Geometry check sheet. Reference: the model listing, model coordinates, mm. Face numbers are marked on the shaded views. A direction names the side the tool comes from. Round coordinates to 2 decimals unless told otherwise and drop trailing zeros. Order: outer loops, then holes, each group sorted by start corner. A loop starts at its lowest first (then second) coordinate and runs counter-clockwise, first axis right, second up.
(1) Release check for a two-part mould opening along Z. For the marked faces 3, 4 and 5 record: +Z half, -Z half, draft (parallel to the pull), parting line (faces both ways), or undercut.
(2) Set-up check for the marked faces 1 and 2: record each of +Z, -Z, +X, -X, +Y, -Y from which the full face is reachable in a straight line by a thin tool's end or side.
(3) Sectioned sample at D-D (x = 30). Record the boundary of the cut face in (y, z).
(4) Sectioned sample at B-B (x = -54). Record the boundary of the cut face in (y, z), plus the area to 3 significant figures.
(5) Sectioned sample at C-C (z = -28.5). Record the boundary of the cut face in (x, y), plus the area to 3 significant figures.
(6) Material ranges on line 1 along Y through (x, z) = (54, -37.65); line 2 along Z through (x, y) = (-28.5, 15.5); line 3 along X through (y, z) = (15.5, 10.5), recorded low to high.
(7) Go/stop test with flat-tipped pins: pin 1 (10 mm diameter, centred on x = 6, z = -13.5, fed in from +Y); pin 2 (6.5 mm diameter, centred on y = 11.5, z = 4, fed in from +X); pin 3 (3 mm diameter, centred on x = -38.5, z = -29, fed in from +Y). Record where each tip stops, or that it passes through.
(8) Sectioned sample at A-A (y = 22). Record the boundary of the cut face in (x, z), plus the area to 3 significant figures.
from build123d import *

# Parameters (mm, degrees)
SKETCH1_W           = 100
SKETCH1_H           = 80
BOSS_EXTRUDE1_DEPTH = 3
SKETCH2_W           = 100
SKETCH2_H           = 80
SKETCH2_W_2         = 97
SKETCH2_H_2         = 77
BOSS_EXTRUDE2_DEPTH = 22
SKETCH3_R           = 1.25
BOSS_EXTRUDE3_DEPTH = 3
CUT_EXTRUDE1_DEPTH  = 3
SKETCH5_W           = 8
SKETCH5_H           = 10.304098564
SKETCH5_R           = 2
BOSS_EXTRUDE4_DEPTH = 5
FILLET8_R           = 1
FILLET9_R           = 1
FILLET10_R          = 1
FILLET11_R          = 1
FILLET12_R          = 1
FILLET13_R          = 1
FILLET14_R          = 1
FILLET15_R          = 1
FILLET16_R          = 1
FILLET17_R          = 1
SKETCH6_W           = 20
SKETCH6_H           = 15
CUT_EXTRUDE2_DEPTH  = 10
FILLET18_R          = 1
FILLET19_R          = 1
FILLET20_R          = 1
FILLET22_R          = 1


with BuildPart() as part:
    # Sketch1 → Boss-Extrude1 (new body)
    with BuildSketch(Plane(origin=(0, 0, 0), x_dir=(1, 0, 0), z_dir=(0, 1, 0))):
        Rectangle(SKETCH1_W, SKETCH1_H)
    extrude(amount=BOSS_EXTRUDE1_DEPTH)

    # Sketch2 → Boss-Extrude2 (add)
    with BuildSketch(Plane(origin=(0, 3, 0), x_dir=(1, 0, 0), z_dir=(0, 1, 0))):
        Rectangle(SKETCH2_W, SKETCH2_H)
        Rectangle(SKETCH2_W_2, SKETCH2_H_2, mode=Mode.SUBTRACT)
    extrude(amount=BOSS_EXTRUDE2_DEPTH)

    # Sketch3 → Boss-Extrude3 (add)
    with BuildSketch(Plane(origin=(0, 3, 0), x_dir=(1, 0, 0), z_dir=(0, 1, 0))):
        with Locations(Location((-38.5, 28.5, 0), (0, 0, 90))):
            Circle(SKETCH3_R)
        with Locations(Location((-38.5, -20.5, 0), (0, 0, 90))):
            Circle(SKETCH3_R)
        with Locations(Location((19.5, 28.5, 0), (0, 0, 90))):
            Circle(SKETCH3_R)
        with Locations(Location((19.5, -20.5, 0), (0, 0, 90))):
            Circle(SKETCH3_R)
    extrude(amount=BOSS_EXTRUDE3_DEPTH)

    # Sketch4 → Cut-Extrude1 (cut)
    with BuildSketch(Plane.XY.offset(40)):
        with BuildLine():
            Line((-33, 15), (-28, 15))
            ThreePointArc((-28, 15), (-23, 10), (-28, 5))
            Line((-28, 5), (-33, 5))
            ThreePointArc((-33, 5), (-38, 10), (-33, 15))
        make_face()
    extrude(amount=-CUT_EXTRUDE1_DEPTH, mode=Mode.SUBTRACT)

    # Sketch5 → Boss-Extrude4 (add)
    # profile 1 of 2: a face of its own
    with BuildSketch(Plane(origin=(0, 0, -40), x_dir=(-1, 0, 0), z_dir=(0, 0, -1))):
        with Locations((54, 11)):
            Rectangle(SKETCH5_W, SKETCH5_H)
        with Locations((54, 11)):
            Circle(SKETCH5_R, mode=Mode.SUBTRACT)
    # profile 2 of 2: a face of its own
    with BuildSketch(Plane(origin=(0, 0, -40), x_dir=(-1, 0, 0), z_dir=(0, 0, -1))):
        with Locations((-54, 11)):
            Rectangle(SKETCH5_W, SKETCH5_H)
        with Locations((-54, 11)):
            Circle(SKETCH5_R, mode=Mode.SUBTRACT)
    extrude(amount=-BOSS_EXTRUDE4_DEPTH)

    # Fillet8
    fillet8_edges = [part.edges().sort_by_distance(p)[0] for p in [
        (58, 16.152049282, -37.5),
    ]]
    fillet(fillet8_edges, radius=FILLET8_R)

    # Fillet9
    fillet9_edges = [part.edges().sort_by_distance(p)[0] for p in [
        (58, 5.847950718, -37.5),
    ]]
    fillet(fillet9_edges, radius=FILLET9_R)

    # Fillet10
    fillet10_edges = [part.edges().sort_by_distance(p)[0] for p in [
        (50, 5.847950718, -37.5),
    ]]
    fillet(fillet10_edges, radius=FILLET10_R)

    # Fillet11
    fillet11_edges = [part.edges().sort_by_distance(p)[0] for p in [
        (50, 16.152049282, -37.5),
    ]]
    fillet(fillet11_edges, radius=FILLET11_R)

    # Fillet12
    fillet12_edges = [part.edges().sort_by_distance(p)[0] for p in [
        (50, 11, -35),
    ]]
    fillet(fillet12_edges, radius=FILLET12_R)

    # Fillet13
    fillet13_edges = [part.edges().sort_by_distance(p)[0] for p in [
        (-58, 5.847950718, -37.5),
    ]]
    fillet(fillet13_edges, radius=FILLET13_R)

    # Fillet14
    fillet14_edges = [part.edges().sort_by_distance(p)[0] for p in [
        (-58, 16.152049282, -37.5),
    ]]
    fillet(fillet14_edges, radius=FILLET14_R)

    # Fillet15
    fillet15_edges = [part.edges().sort_by_distance(p)[0] for p in [
        (-50, 5.847950718, -37.5),
    ]]
    fillet(fillet15_edges, radius=FILLET15_R)

    # Fillet16
    fillet16_edges = [part.edges().sort_by_distance(p)[0] for p in [
        (-50, 16.152049282, -37.5),
    ]]
    fillet(fillet16_edges, radius=FILLET16_R)

    # Fillet17
    fillet17_edges = [part.edges().sort_by_distance(p)[0] for p in [
        (-50, 11, -35),
    ]]
    fillet(fillet17_edges, radius=FILLET17_R)

    # Sketch6 → Cut-Extrude2 (cut)
    with BuildSketch(Plane(origin=(50, 0, 0), x_dir=(0, 0, -1), z_dir=(1, 0, 0))):
        with Locations((4.6, 9.5)):
            Rectangle(SKETCH6_W, SKETCH6_H)
    extrude(amount=-CUT_EXTRUDE2_DEPTH, mode=Mode.SUBTRACT)

    # Fillet18
    fillet18_edges = [part.edges().sort_by_distance(p)[0] for p in [
        (45, 2, 5.4),
    ]]
    fillet(fillet18_edges, radius=FILLET18_R)

    # Fillet19
    fillet19_edges = [part.edges().sort_by_distance(p)[0] for p in [
        (45, 2, -14.6),
    ]]
    fillet(fillet19_edges, radius=FILLET19_R)

    # Fillet20
    fillet20_edges = [part.edges().sort_by_distance(p)[0] for p in [
        (49.25, 17, 5.4),
    ]]
    fillet(fillet20_edges, radius=FILLET20_R)

    # Fillet22
    fillet22_edges = [part.edges().sort_by_distance(p)[0] for p in [
        (49.25, 17, -14.6),
    ]]
    fillet(fillet22_edges, radius=FILLET22_R)


solid = part.part
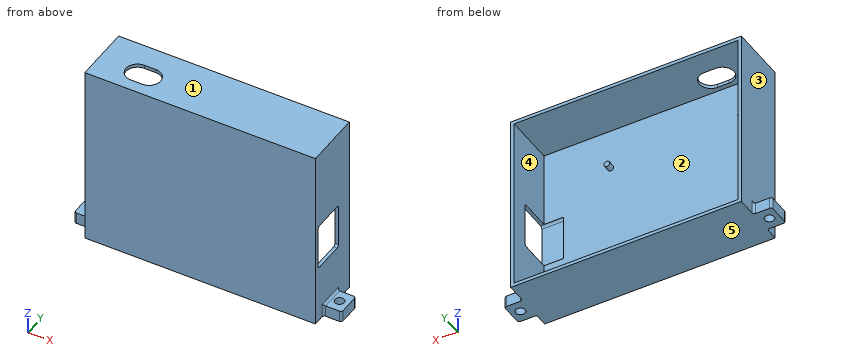
Answer below:
1. face 3: draft
1. face 4: undercut
1. face 5: -Z half
2. face 1: +Z, +X, -X, +Y, -Y
2. face 2: +Y
3. outline: (0, -40) - (25, -40) - (25, -38.5) - (3, -38.5) - (3, 38.5) - (25, 38.5) - (25, 40) - (0, 40) - close
4. outline: (5.85, -40) - (9, -40) - (9, -35) - (5.85, -35) - close; (13, -40) - (16.15, -40) - (16.15, -35) - (13, -35) - close
4. area: 31.5 mm2
5. outline: (-50, 0) - (50, 0) - (50, 25) - (48.5, 25) - (48.5, 3) - (20.75, 3) - (20.75, 6) - (18.25, 6) - (18.25, 3) - (-37.25, 3) - (-37.25, 6) - (-39.75, 6) - (-39.75, 3) - (-48.5, 3) - (-48.5, 25) - (-50, 25) - close
5. area: 381 mm2
6. line 1: y = 5.85 to 9, 13 to 16.15
6. line 2: z = -40 to -38.5, 38.5 to 40
6. line 3: x = -50 to -48.5, 48.5 to 50
7. pin 1: stops at y = 3
7. pin 2: stops at x = 50
7. pin 3: stops at y = 6
8. outline: (-50, -40) - (50, -40) - (50, 40) - (-50, 40) - close; hole (-48.5, -38.5) - (48.5, -38.5) - (48.5, 38.5) - (-48.5, 38.5) - close
8. area: 531 mm2
